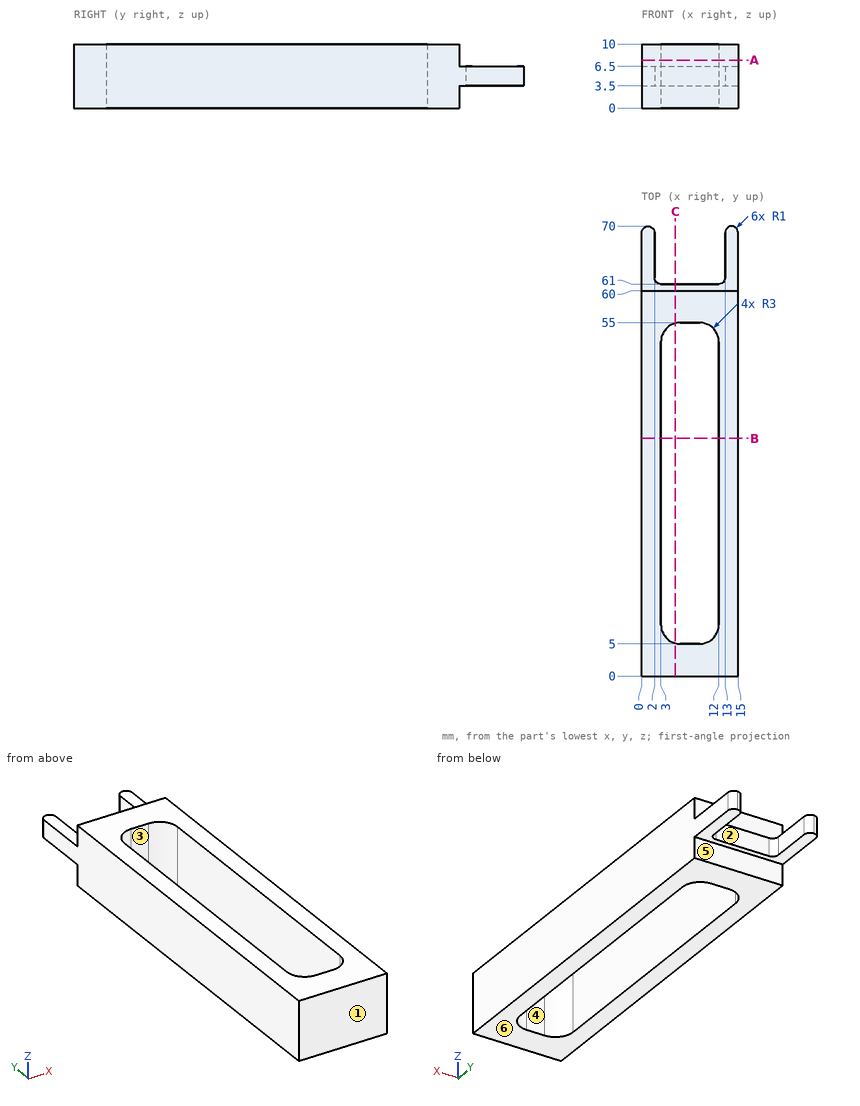
For this review, use the dimensioned drawing (mm, ordinates from the lowest corner) and the shaded views. A direction names the side the tool comes from. Round coordinates to 2 decimals unless told otherwise and drop trailing zeros. Write each loop counter-clockwise with the first axis right and the second up, starting at its lowest first coordinate (ties: lowest second). Pieces come first, ordered by that corner, then holes. Notation, with made-up numbers: M -7,20.5 L 0,20.5 A9 cw 0,32.5 Z; hole C 7,-18.75 d7. An arc over 180 degrees is marked long. Use CSV: the item, a comma, the result in double quotes. Start each with the question number.
(1) We need section A-A, the plane z = 7.5. State the section outline as (x, y) points, then the cut area to 3 significant figures.
(2) For line 1 along Y through (x, z) = (9.25, 1); line 2 along X through (y, z) = (48, 5.5); line 3 along Y through (x, z) = (12.25, 1.75), list the stretches that pass through material, from the lowest coordinate up.
(3) We need section B-B, the plane y = 37. State the section outline as (x, z) points, then the cut area to 3 significant figures.
(4) The part is to be moulded in two halves that separate along Y. For the marked faces 4, 5 and 6, say which applies: +Y half, -Y half, draft (parallel to the pull), parting line (faces both ways), or undercut.
(5) We need section C-C, the plane x = 5.25. State the section outline as (y, z) points.
(6) Tool access review of the marked faces 1, 2 and 3: name each direction out of +Z, -Z, +X, -X, +Y, -Y from which nothing blocks a thin tool from reaching the whole face with its end or side.
(7) Clearance check with flat-ended pins moving along their axes: P1, Ø1, axis at x = 6.5, z = 8.5, coming from the +Y side; P2, Ø1.5, axis at x = 8.5, z = 4.5, coming from the +Y side; P3, Ø8, axis at x = 10.5, y = 65, coming from the -Z side. State where each tip first meets the part, or that it passes through.
Findings:
1,outline,"M 0,0 L 15,0 L 15,60 L 0,60 Z; hole M 3,8 A3 ccw 6,5 L 9,5 A3 ccw 12,8 L 12,52 A3 ccw 9,55 L 6,55 A3 ccw 3,52 Z"
1,area,"458 mm^2"
2,line 1,"0 to 5.01, 54.99 to 60"
2,line 2,"0 to 3, 12 to 15"
2,line 3,"0 to 60"
3,outline,"M 0,0 L 3,0 L 3,10 L 0,10 Z; M 12,0 L 15,0 L 15,10 L 12,10 Z"
3,area,"60.0 mm^2"
4,face 4,"undercut"
4,face 5,"+Y half"
4,face 6,"draft"
5,outline,"M 0,0 L 5.1,0 L 5.1,10 L 0,10 Z; M 54.9,0 L 60,0 L 60,3.5 L 61,3.5 L 61,6.5 L 60,6.5 L 60,10 L 54.9,10 Z"
6,face 1,"+Z, -Z, +X, -X, -Y"
6,face 2,"+Z, -Z, +Y"
6,face 3,"+Z, -Z"
7,P1,"y = 60"
7,P2,"y = 61"
7,P3,"z = 3.5"
